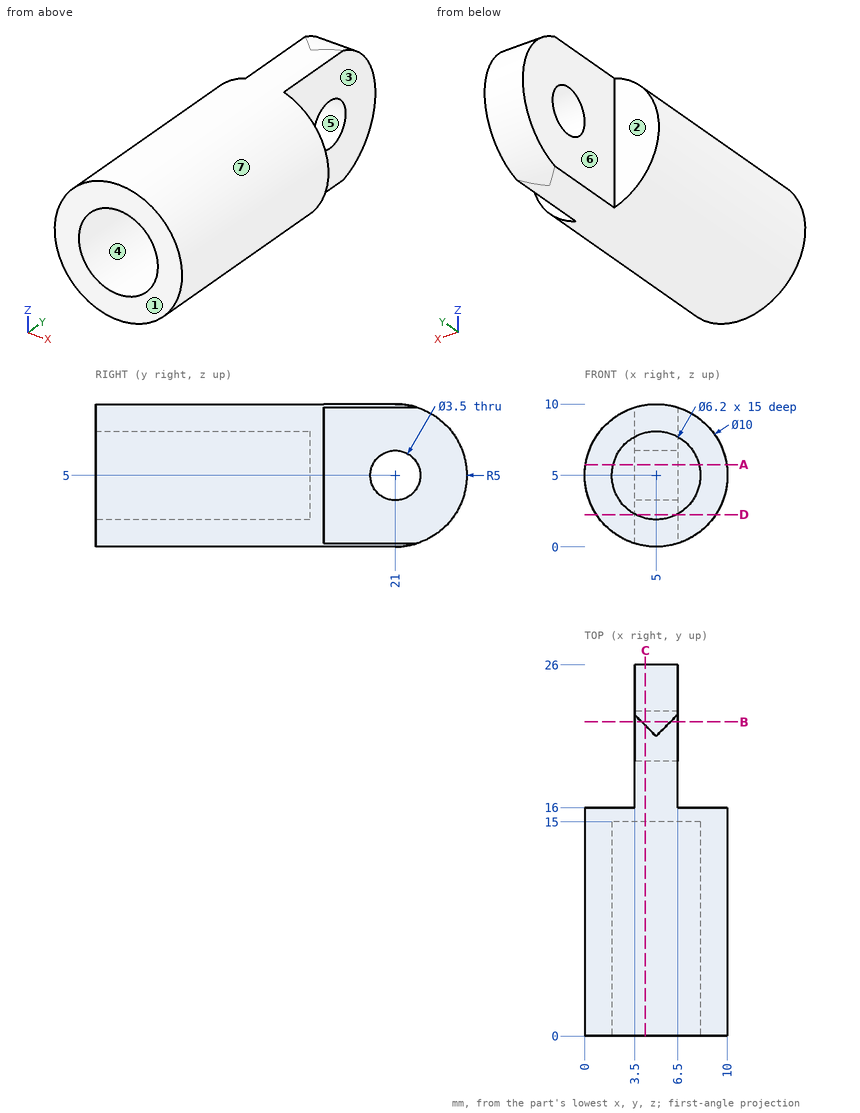
Here's the drawing with two shaded views (mm, measured from the low corner). I have some questions. A direction names the side the tool comes from. Coordinates: 2 decimals unless noted, no trailing zeros. Loops run counter-clockwise (first coordinate to the right, second up) from the corner with the lowest first, then second, coordinate; pieces in that order, holes last. Notation, with made-up numbers: M 79,26 L 98,26 A17 ccw 98,34 Z; hole C 48.5,35 d9. An arc over 180 degrees is marked long. Return JSON: item names as keys, results as strings. Group by question number.
Item 1: Thinking about a two-plate mould opening in X: for the marked faces 4, 5, 6 and 7, which applies, released by +X, released by -X, zero draft, split by the parting line, or undercut?
Item 2: Imagine slicing it at A-A (z = 5.75). Please give me the cut outline in (x, y).
Item 3: Imagine slicing it at B-B (y = 22). Please give me the cut outline in (x, z).
Item 4: If I drill on L1, parallel to Y at x = 4.7, z = 5; L2, parallel to X at y = 12, z = 5; L3, parallel to Y at x = 1.75, z = 5.5, over which ranges is the centre line in solid material (lowest first)? Write a range as from..to.
Item 5: Imagine slicing it at C-C (x = 4.25). Please give me the cut outline in (y, z).
Item 6: I'm going to push flat-ended pins straight in: pin 1 Ø4 at (x, y) = (3, 22.5) entering from -Z; pin 2 Ø1 at (x, z) = (2.5, 6) entering from +Y; pin 3 Ø6 at (x, y) = (4, 17) entering from +Z; pin 4 Ø5 at (y, z) = (9.5, 8.5) entering from -X. Where does each tip first touch, or does it pass through?
Item 7: Imagine slicing it at D-D (z = 2.25). Please give me the cut outline in (x, y), and give its area (3 significant figures).
Item 8: On a 3-axis mill with a long thin cutter (end or side, diameter ignored), from which of +Z, -Z, +X, -X, +Y, -Y can I reach the whole of each face in a straight line? I mean the marked faces 1, 2 and 3. Say none if no direction works.
Verdict:
{
 "1": {"face 4": "undercut", "face 5": "zero draft", "face 6": "released by -X", "face 7": "split by the parting line"},
 "2": {"outline": "M 0.06,0 L 1.99,0 L 1.99,15 L 8.01,15 L 8.01,0 L 9.94,0 L 9.94,16 L 6.5,16 L 6.5,19.42 L 3.5,19.42 L 3.5,16 L 0.06,16 Z; M 3.5,22.58 L 6.5,22.58 L 6.5,25.94 L 3.5,25.94 Z"},
 "3": {"outline": "M 3.5,0.23 A5 ccw 4,0.1 L 6,0.1 A5 ccw 6.5,0.23 L 6.5,3.56 L 3.5,3.56 Z; M 3.5,6.44 L 6.5,6.44 L 6.5,9.77 A5 ccw 6,9.9 L 4,9.9 A5 ccw 3.5,9.77 Z"},
 "4": {"L1": "y = 15..19.25, 22.75..26", "L2": "x = 0..1.9, 8.1..10", "L3": "y = 0..16"},
 "5": {"outline": "M 0,0.06 L 21.75,0.06 A5 ccw 21.75,9.94 L 0,9.94 L 0,8.01 L 15,8.01 L 15,1.99 L 0,1.99 Z; hole C 21,5 d3.5"},
 "6": {"pin 1": "stops at z = 0.01", "pin 2": "stops at y = 16", "pin 3": "stops at z = 10", "pin 4": "stops at x = 0.1"},
 "7": {"outline": "M 0.82,0 L 3.57,0 L 3.57,15 L 6.43,15 L 6.43,0 L 9.18,0 L 9.18,16 L 6.5,16 L 6.5,25.18 L 3.5,25.18 L 3.5,16 L 0.82,16 Z", "area": "118 mm^2"},
 "8": {"face 1": "+Z, -Z, +X, -X, -Y", "face 2": "+Z, -Z, -X, +Y", "face 3": "+Z, -Z, +X, +Y"}
}
